Check sheet for the modelled part. Datum: model origin and axes. Units: mm. Coordinates: 2 decimals unless noted, no trailing zeros. Loops run counter-clockwise (first coordinate to the right, second up) from the corner with the lowest first, then second, coordinate; pieces in that order, holes last. Notation, with made-up numbers: M 17,75 L 28,75 A28 ccw 28,104 Z; hole C 83.5,-29 d11. An arc over 180 degrees is marked long. Return JSON: item names as keys, results as strings.
Autodesk Inventor part; units mm, degrees
ref_plane "YZ Plane" through (0, 0, 0) normal (1, 0, 0) x (0, 1, 0)
ref_plane "XZ Plane" through (0, 0, 0) normal (0, 1, 0) x (-1, 0, 0)
ref_plane "XY Plane" through (0, 0, 0) normal (0, 0, 1) x (1, 0, 0)
sketch "Sketch1" plane through (0, 0, 0) normal (0, 1, 0) x (-1, 0, 0)
  line L0 (-25.425, 54.65) -> (25.425, 54.65)
  line L1 (25.425, 54.65) -> (25.425, -54.65)
  line L2 (25.425, -54.65) -> (-25.425, -54.65)
  line L3 (-25.425, -54.65) -> (-25.425, 54.65)
  line L4 (-25.425, 54.65) -> (25.425, -54.65) construction
  line L5 (25.425, 54.65) -> (-25.425, -54.65) construction
  point P0 (0, 0)
  dimension "d0" = 109.3
  dimension "d1" = 50.85
extrude "Extrusion1" add sketch "Sketch1" along normal blind 185
shell "Shell1" thickness 1 removed faces 1 at (8.475, 0, 18.2167)
sketch "Sketch2" plane through (0, 0, 0) normal (0, -1, 0) x (1, 0, 0)
  line L0 (-24.425, -53.65) -> (-24.425, 53.65)
  line L1 (-24.425, 53.65) -> (24.425, 53.65)
  line L2 (24.425, 53.65) -> (24.425, -53.65)
  line L3 (24.425, -53.65) -> (-24.425, -53.65)
  line L4 (25.425, 54.65) -> (-25.425, 54.65)
  line L5 (-25.425, 54.65) -> (-25.425, -54.65)
  line L6 (-25.425, -54.65) -> (25.425, -54.65)
  line L7 (25.425, -54.65) -> (25.425, 54.65)
  line L8 (-24.425, 53.65) -> (-24.425, 54.65)
  line L9 (25.425, 54.65) -> (-25.425, 54.65)
  line L10 (24.425, 53.65) -> (24.425, -53.65)
  line L11 (24.425, -53.65) -> (25.425, -53.65)
  line L12 (25.425, -54.65) -> (25.425, 54.65)
  point P0 (0, 0)
extrude "Extrusion2" add sketch "Sketch2" along normal blind 10.9 contours L3 L11 L7 L6 L5 L4 L8 L0
sketch "Sketch3" plane through (25.425, 185, -54.65) normal (0, 0, -1) x (-1, 0, 0)
  line L0 (0, -176.75) -> (50.85, -176.75) construction
  line L1 (50.85, 0) -> (50.85, -195.9) construction
  circle A0 centre (25.425, -176.75) radius 1.5
  line L2 (50.85, -195.9) -> (0, -195.9)
  line L3 (0, 0) -> (0, -195.9)
  line L4 (25.425, -176.75) -> (25.425, -38.45) construction
  circle A1 centre (25.425, -38.45) radius 1.5
  line L5 (25.425, -38.45) -> (39.825, -38.45) construction
  line L6 (39.825, -38.45) -> (39.825, -17.85) construction
  circle A2 centre (39.825, -17.85) radius 1.5
  point P0 (25.425, -185)
  dimension "d7" = 19.15
  dimension "d8" = 3
  dimension "d9" = 138.3
  dimension "d10" = 3
  dimension "d11" = 14.4
  dimension "d12" = 20.6
  dimension "d13" = 3
extrude "Extrusion3" cut sketch "Sketch3" against normal up to surface (1 mm away)
sketch "Sketch4" plane through (-25.425, 185, -54.65) normal (-1, 0, 0) x (0, 0, 1)
  line L0 (0, -191.45) -> (109.3, -191.45) construction
  line L1 (109.3, 0) -> (109.3, -195.9) construction
  line L2 (109.3, -195.9) -> (0, -195.9) construction
  line L3 (0, 0) -> (0, -195.9) construction
  circle A0 centre (6.3, -191.45) radius 1.5
  circle A1 centre (102.3, -191.45) radius 1.5
  line L4 (0, -134.85) -> (109.3, -134.85) construction
  circle A2 centre (14.75, -134.85) radius 1.5
  circle A3 centre (99.8, -134.85) radius 1.5
  line L5 (0, -18.65) -> (109.3, -18.65) construction
  circle A4 centre (102.6, -18.65) radius 1.5
  line L6 (0, -8.85) -> (109.3, -8.85) construction
  circle A5 centre (14.6, -8.85) radius 1.5
  circle A6 centre (99.4, -8.85) radius 1.5
  point P0 (54.65, -185)
  dimension "d16" = 4.45
  dimension "d17" = 7
  dimension "d18" = 3
  dimension "d19" = 6.3
  dimension "d20" = 3
  dimension "d21" = 56.6
  dimension "d22" = 14.75
  dimension "d23" = 9.5
  dimension "d24" = 3
  dimension "d25" = 3
  dimension "d26" = 116.2
  dimension "d27" = 6.7
  dimension "d28" = 3
  dimension "d29" = 9.8
  dimension "d30" = 9.9
  dimension "d31" = 3
  dimension "d32" = 14.6
  dimension "d33" = 3
extrude "Extrusion4" cut sketch "Sketch4" against normal up to surface (1 mm away)
ref_plane "Work Plane1" through (-19.425, 0, 53.65) normal (1, 0, 0) x (0, 0, -1)
sketch "Sketch5" plane through (-19.425, 0, 53.65) normal (1, 0, 0) x (0, 0, -1)
  line L0 (107.3, -10.9) -> (-1, -10.9)
  line L1 (97.3, -10.9) -> (97.3, 0)
  line L2 (107.3, 0) -> (107.3, -10.9)
  line L3 (11, -10.9) -> (11, 0)
  line L4 (-1, 0) -> (-1, -10.9)
  line L5 (11, -10.9) -> (97.3, -10.9)
  line L6 (11, 0) -> (-1, 0)
  line L7 (-1, 185) -> (-1, -10.9)
  line L8 (97.3, 0) -> (107.3, 0)
  line L9 (107.3, -10.9) -> (107.3, 184)
  line L10 (-1, 0) -> (11, 0)
  line L11 (0, 0) -> (0, 184)
  line L12 (0, 0) -> (0, 50)
  line L13 (0, 50) -> (107.3, 50)
  line L14 (107.3, 50) -> (107.3, 0)
  point P0 (53.65, 0)
  dimension "d36" = 10
  dimension "d37" = 12
  dimension "d38" = 50
extrude "Extrusion5" add sketch "Sketch5" along normal blind 1.5 contours L0 L3 L6 L11 L13 L9 L8 L1
sketch "Sketch6" plane through (-17.925, 0, 53.65) normal (1, 0, 0) x (0, 0, -1)
  line L0 (97.3, 0) -> (107.3, 0)
  line L1 (97.3, 0) -> (11, 0)
  line L2 (11, 0) -> (11, -11.9)
  line L3 (11, -11.9) -> (97.3, -11.9)
  line L4 (97.3, -11.9) -> (97.3, 0)
  line L5 (11, 0) -> (11, -10.9)
  line L6 (11, -10.9) -> (97.3, -10.9)
  point P0 (53.65, 0)
  dimension "d42" = 1
extrude "Extrusion6" add sketch "Sketch6" along normal blind 16
sketch "Sketch7" plane through (-17.925, -11.9, -43.65) normal (0, -1, 0) x (1, 0, 0)
  line L0 (13.5, 84.8) -> (8.5, 84.8)
  line L1 (8.5, 84.8) -> (8.5, 57.8)
  line L2 (8.5, 57.8) -> (13.5, 57.8)
  line L3 (13.5, 57.8) -> (13.5, 84.8)
  line L4 (0, 86.3) -> (16, 86.3)
  line L5 (16, 86.3) -> (16, 0)
  line L6 (0, 86.3) -> (0, 0)
  line L7 (13.5, 56.3) -> (8.5, 56.3)
  line L8 (8.5, 56.3) -> (8.5, 1.5)
  line L9 (8.5, 1.5) -> (13.5, 1.5)
  line L10 (13.5, 1.5) -> (13.5, 56.3)
  line L11 (0, 0) -> (16, 0)
  point P0 (17.925, 43.65)
  dimension "d45" = 1.5
  dimension "d46" = 2.5
  dimension "d47" = 27
  dimension "d48" = 8.5
  dimension "d49" = 1.5
  dimension "d50" = 1.5
extrude "Extrusion7" cut sketch "Sketch7" against normal blind 16 contours L3 L2 L1 L0 | L10 L9 L8 L7
ref_plane "Work Plane2" through (0, -35.9, 0) normal (0, -1, 0) x (1, 0, 0)
ref_plane "Work Plane3" through (-25.425, 185, 0) normal (0, 0, 1) x (1, 0, 0)
properties part number "PSU"
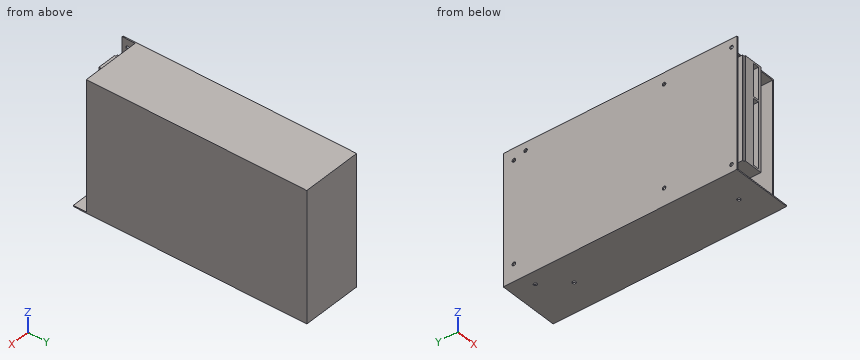
1) Section check B-B on x = 19.5. Record the cut outline in (y, z).
Answers:
{"outline": "M -10.9,-54.65 L 185,-54.65 L 185,54.65 L 0,54.65 L 0,53.65 L 184,53.65 L 184,-53.65 L -10.9,-53.65 Z"}
2) Go/stop test with flat-tipped pins: pin 1 Ø1.2 at (x, z) = (-18.5, -48.5) entering from -Y; pin 2 Ø5.5 at (x, y) = (-6.5, -6.5) entering from +Z; pin 3 Ø0.5 at (y, z) = (-11.5, 5) entering from -X (3 decimals); pin 4 Ø1.6 at (x, z) = (-18.5, -0.5) entering from -Y. Record where each tip stops, or that it passes through.
Answers:
{"pin 1": "y = 0", "pin 2": "z = 42.65", "pin 3": "x = -17.925", "pin 4": "y = -11.9"}
3) Section check A-A on z = 29. Record the cut outline in (x, y) (3 decimals).
Answers:
{"outline": "M -25.425,-10.9 L -24.425,-10.9 L -24.425,184 L 24.425,184 L 24.425,0 L 25.425,0 L 25.425,185 L -25.425,185 Z; M -19.425,-10.9 L -17.925,-10.9 L -17.925,-11.9 L -9.425,-11.9 L -9.425,0 L -17.925,0 L -17.925,50 L -19.425,50 Z; M -4.425,-11.9 L -1.925,-11.9 L -1.925,0 L -4.425,0 Z"}
4) Scan lines: line 1 along Y through (x, z) = (0, -54); line 2 along Y through (x, z) = (-24.8, 47.65); line 3 along X through (y, z) = (15.5, 9.5) (3 decimals). Record each from-to range of solid material in increasing order. Write a range as [from, to].
Answers:
{"line 1": "[-10.9, 6.75], [9.75, 145.05], [148.05, 185]", "line 2": "[-10.9, -7.95], [-4.95, 164.88], [167.82, 185]", "line 3": "[-25.425, -24.425], [-19.425, -17.925], [24.425, 25.425]"}
